Can you work these out from the model? Positions are in its coordinate system, mm. Face numbers are marked on the shaded views. A direction names the side the tool comes from. Give positions to 0.01 mm unless a question says otherwise; leave off trailing zeros. Loops run counter-clockwise (first coordinate to the right, second up) from the corner with the lowest first, then second, coordinate; pieces in that order, holes last. Notation, with made-up numbers: M 65.25,44.5 L 103.25,44.5 A17 ccw 103.25,53.5 Z; hole C 20,34.25 d11. An arc over 180 degrees is marked long. Put each result on its own line as item: value. Start each with the question number.
1) Please list where these lines run through material, in increasing order: line 1 along Z through (x, y) = (-17.5, 2); line 2 along X through (y, z) = (-4, -90.5); line 3 along X through (y, z) = (-3, -91). Write a range as from..to.
2) Imagine slicing it at C-C (z = -92). Write out the boundary of the cut face in (x, y).
3) For P1, Ø4, axis at y = 3, z = -34.5, coming from the +X side; P2, Ø3, axis at y = 3.5, z = -61.5, coming from the -X side; P3, Ø6.5, axis at x = 0, y = 12.5, coming from the +Z side; P4, Ø5, axis at x = 8, z = -74.5, coming from the -Y side, each with a flat end and sliding along its axis, tell me the tip position at first contact or that it passes through.
4) Imagine slicing it at A-A (z = -37.5). Write out the boundary of the cut face in (x, y), then the cut area to 3 significant figures.
5) For the marked faces 1 and 2, which set-ups out of +Z, -Z, +X, -X, +Y, -Y let a thin tool reach every point of the face, with its end or its side?
6) Imagine slicing it at B-B (y = -7). Write out the boundary of the cut face in (x, z) (3 decimals).
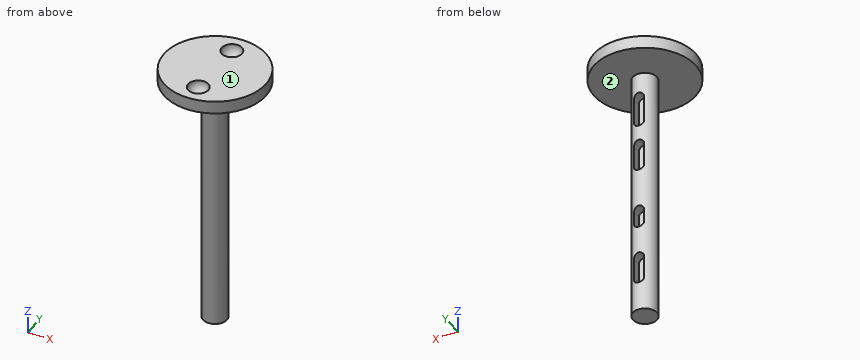
from build123d import *

# Parameters (mm, degrees)
SKETCH1_R           = 20
BOSS_EXTRUDE1_DEPTH = 5
SKETCH3_R           = 4
CUT_EXTRUDE2_DEPTH  = 4
FILLET2_R           = 4
SKETCH4_R           = 4.75
BOSS_EXTRUDE2_DEPTH = 105
CUT_EXTRUDE3_DEPTH  = 4
CUT_EXTRUDE4_START  = -5
SKETCH6_R           = 4.75
CUT_EXTRUDE4_DEPTH  = 5


with BuildPart() as part:
    # Sketch1 → Boss-Extrude1 (new body)
    with BuildSketch(Plane.XY):
        Circle(SKETCH1_R)
    extrude(amount=BOSS_EXTRUDE1_DEPTH)

    # Sketch3 → Cut-Extrude2 (cut)
    with BuildSketch(Plane.XY.offset(5)):
        with Locations((0, 12.5)):
            Circle(SKETCH3_R)
        with Locations((0, -12.5)):
            Circle(SKETCH3_R)
    extrude(amount=-CUT_EXTRUDE2_DEPTH, mode=Mode.SUBTRACT)

    # Fillet2
    fillet2_edges = [part.edges().sort_by_distance(p)[0] for p in [
        (-4, 12.5, 1),
        (-4, -12.5, 1),
    ]]
    fillet(fillet2_edges, radius=FILLET2_R - 0.0001)  # a hair under: the kernel refuses the full size

    # Sketch4 → Boss-Extrude2 (add)
    with BuildSketch(Plane(origin=(0, 0, 0), x_dir=(-1, 0, 0), z_dir=(0, 0, -1))):
        Circle(SKETCH4_R)
    extrude(amount=BOSS_EXTRUDE2_DEPTH)

    # Sketch5 → Cut-Extrude3 (cut)
    with BuildSketch(Plane(origin=(0, 4.75, 0), x_dir=(1, 0, 0), z_dir=(0, 1, 0))):
        with BuildLine():
            Line((-2, 10), (-2, 20))
            ThreePointArc((-2, 20), (0, 22), (2, 20))
            Line((2, 20), (2, 10))
            ThreePointArc((2, 10), (0, 8), (-2, 10))
        make_face()
        with BuildLine():
            Line((-2, 30), (-2, 38.71))
            ThreePointArc((-2, 38.71), (0, 40.71), (2, 38.71))
            Line((2, 38.71), (2, 30))
            ThreePointArc((2, 30), (0, 28), (-2, 30))
        make_face()
        with BuildLine():
            Line((-2, 77.83), (-2, 86.54))
            ThreePointArc((-2, 86.54), (0, 88.54), (2, 86.54))
            Line((2, 86.54), (2, 77.83))
            ThreePointArc((2, 77.83), (0, 75.83), (-2, 77.83))
        make_face()
        with BuildLine():
            Line((-2, 57.92), (-2, 62.92))
            ThreePointArc((-2, 62.92), (0, 64.92), (2, 62.92))
            Line((2, 62.92), (2, 57.92))
            ThreePointArc((2, 57.92), (0, 55.92), (-2, 57.92))
        make_face()
    extrude(amount=-CUT_EXTRUDE3_DEPTH, mode=Mode.SUBTRACT)

    # Sketch6 → Cut-Extrude4 (cut)
    with BuildSketch(Plane(origin=(0, 0, -105), x_dir=(-1, 0, 0), z_dir=(0, 0, -1)).offset(CUT_EXTRUDE4_START)):
        Circle(SKETCH6_R)
    extrude(amount=CUT_EXTRUDE4_DEPTH, mode=Mode.SUBTRACT)


solid = part.part
Recorded:
1. line 1: 0..5
1. line 2: -2.56..2.56
1. line 3: -3.68..3.68
2. outline: C 0,0 d9.5
3. P1: x = 4.64
3. P2: x = -4.31
3. P3: z = 2.67
3. P4: through
4. outline: M -2,0.75 L -2,4.31 A4.75 ccw long 2,4.31 L 2,0.75 Z
4. area: 55.5 mm²
5. face 1: +Z, +X, -X, +Y, -Y
5. face 2: -Z
6. outline: M -18.735,0 L 18.735,0 L 18.735,5 L -18.735,5 Z
